Geometry check sheet. Reference: drawing and pictorial views, mm from the part's lowest x, y, z. A direction names the side the tool comes from. Round coordinates to 2 decimals unless told otherwise and drop trailing zeros. Write each loop counter-clockwise with the first axis right and the second up, starting at its lowest first coordinate (ties: lowest second). Pieces come first, ordered by that corner, then holes. Notation, with made-up numbers: (21, 89) - (75, 89) arc R21 ccw to (75, 113) - close; hole circle Ø4 at (-32.5, 5.5). An arc over 180 degrees is marked (long way). Return JSON: item names as keys, results as strings.
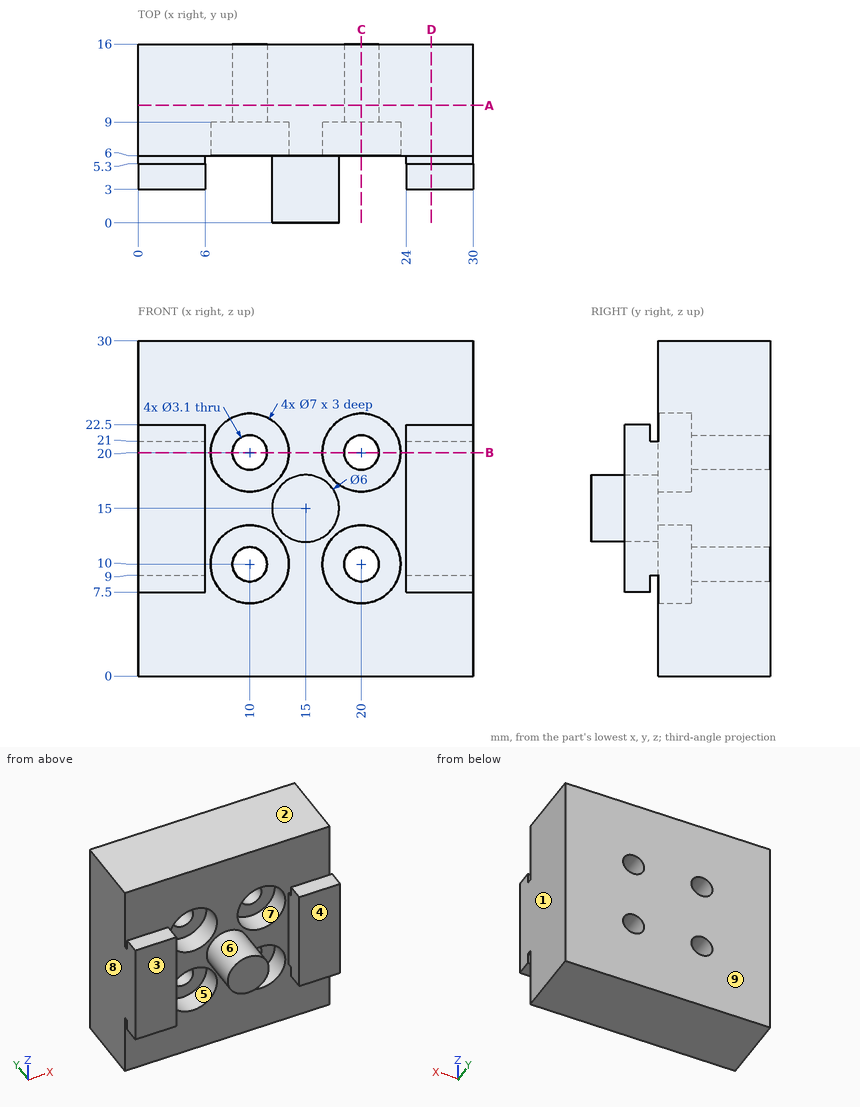
(1) Section check D-D, the plane x = 26.25. Enter the section's corners in (y, z), plus the area to 3 significant figures.
Response values:
{"outline": "(3, 7.5) - (5.3, 7.5) - (5.3, 9) - (6, 9) - (6, 0) - (16, 0) - (16, 30) - (6, 30) - (6, 21) - (5.3, 21) - (5.3, 22.5) - (3, 22.5) - close", "area": "343 mm^2"}
(2) Material ranges on line 1 along Z through (x, y) = (20, 11); line 2 along X through (y, z) = (7.5, 10), recorded low to high. Write a range as [from, to].
Response values:
{"line 1": "z = [0, 8.45], [11.55, 18.45], [21.55, 30]", "line 2": "x = [0, 6.5], [13.5, 16.5], [23.5, 30]"}
(3) Access from +Z, -Z, +X, -X, +Y, -Y to the whole of each face (thin tool, end or side, straight path). Record for the marked faces 1, 2, 3, 4 and 5.
Response values:
{"face 1": "+Z, -Z, +X, +Y, -Y", "face 2": "+Z, +X, -X, +Y, -Y", "face 3": "+Z, -Z, -X, -Y", "face 4": "+Z, -Z, +X, -Y", "face 5": "-Y"}
(4) Section check A-A, the plane y = 10.5. Enter the section's corners in (x, z).
Response values:
{"outline": "(0, 0) - (30, 0) - (30, 30) - (0, 30) - close; hole circle Ø3.1 at (10, 10); hole circle Ø3.1 at (10, 20); hole circle Ø3.1 at (20, 10); hole circle Ø3.1 at (20, 20)"}
(5) Gauge pin test, flat ends, axial feed: pin 1 (6 mm diameter, centred on x = 20, z = 8, fed in from -Y); pin 2 (2.5 mm diameter, centred on x = 4, y = 4.5, fed in from -Z); pin 3 (3.5 mm diameter, centred on x = 18.5, z = 20, fed in from -Y); pin 4 (1.9 mm diameter, centred on x = 10, z = 20, fed in from +Y) (3 decimals). Record the tip position at first contact, or that the pin passes through.
Response values:
{"pin 1": "stops at y = 6", "pin 2": "stops at z = 7.5", "pin 3": "stops at y = 9", "pin 4": "passes through"}
(6) Section check B-B, the plane z = 20. Enter the section's corners in (x, y), plus the area to 3 significant figures.
Response values:
{"outline": "(0, 3) - (6, 3) - (6, 6) - (6.5, 6) - (6.5, 9) - (8.45, 9) - (8.45, 16) - (0, 16) - close; (11.55, 9) - (13.5, 9) - (13.5, 6) - (16.5, 6) - (16.5, 9) - (18.45, 9) - (18.45, 16) - (11.55, 16) - close; (21.55, 9) - (23.5, 9) - (23.5, 6) - (24, 6) - (24, 3) - (30, 3) - (30, 16) - (21.55, 16) - close", "area": "251 mm^2"}
(7) Section check C-C, the plane x = 20. Enter the section's corners in (y, z), plus the area to 3 significant figures.
Response values:
{"outline": "(6, 0) - (16, 0) - (16, 8.45) - (9, 8.45) - (9, 6.5) - (6, 6.5) - close; (6, 13.5) - (9, 13.5) - (9, 11.55) - (16, 11.55) - (16, 18.45) - (9, 18.45) - (9, 16.5) - (6, 16.5) - close; (6, 23.5) - (9, 23.5) - (9, 21.55) - (16, 21.55) - (16, 30) - (6, 30) - close", "area": "215 mm^2"}
(8) Release check for a two-part mould opening along X. For the marked faces 6, 7, 8 and 9 record: pulls with the +X half, pulls with the -X half, needs draft (parallel to the pull), parting line crosses it, or undercut.
Response values:
{"face 6": "undercut", "face 7": "undercut", "face 8": "pulls with the -X half", "face 9": "needs draft"}
